Build history of the part. All positions in model axes, mm. Round coordinates to 2 decimals unless told otherwise and drop trailing zeros. Order: outer loops, then holes, each group sorted by start corner. A loop starts at its lowest first (then second) coordinate and runs counter-clockwise, first axis right, second up. Notation, with made-up numbers: M 8,39 L 37,39 A23 cw 37,58 Z; hole C 13.25,54.5 d11. An arc over 180 degrees is marked long. Use CSV: the item, a comma, the result in double quotes.
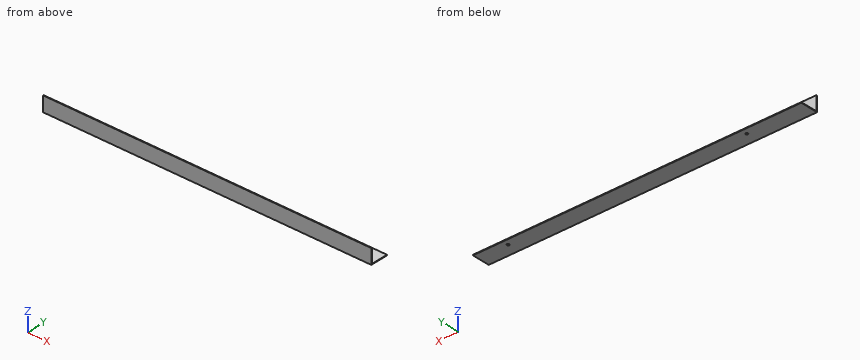
from build123d import *

# Parameters (mm, degrees)
F0_W     = 550
F0_H     = 30
F1_DEPTH = 1
F2_W     = 550
F2_H     = 1
F3_DEPTH = 24
F4_R     = 2
F5_DEPTH = 1.001


with BuildPart() as f1:
    # F0 (on Top) → F1 (new body)
    with BuildSketch(Plane.XY):
        with Locations((275, 15)):
            Rectangle(F0_W, F0_H)
    extrude(amount=F1_DEPTH)

    # F2 (on face) → F3 (join)
    with BuildSketch(Plane.XY.offset(1)):
        with Locations((275, 0.5)):
            Rectangle(F2_W, F2_H)
    extrude(amount=F3_DEPTH)

    # F4 (on face) → F5 (cut, through all)
    with BuildSketch(Plane.XY.offset(1)):
        with Locations((100, 20)):
            Circle(F4_R)
        with Locations((500, 20)):
            Circle(F4_R)
    extrude(amount=-F5_DEPTH, mode=Mode.SUBTRACT)


solid = f1.part
(1) Cut at B-B, the plane z = 14.75. Give the cut face in (x, y), and give its area (3 significant figures).
Answer block:
outline,"M 0,0 L 550,0 L 550,1 L 0,1 Z"
area,"550 mm²"
(2) Drop flat-ended pins along their axis: pin 1 (14.5 mm diameter, centred on x = 403, y = 16, fed in from +Z); pin 2 (2 mm diameter, centred on x = 271.5, z = 5.5, fed in from +Y). Give the stop position or say it passes through.
Answer block:
pin 1,"stops at z = 1"
pin 2,"stops at y = 1"
(3) Cut at A-A, the plane x = 188.5. Give the cut face in (y, z), and give its area (3 significant figures).
Answer block:
outline,"M 0,0 L 30,0 L 30,1 L 1,1 L 1,25 L 0,25 Z"
area,"54.0 mm²"
(4) Wall check: line 1 (Y direction, x = 100, z = 0.25); line 2 (Y direction, x = 235.5, z = 10.75). Give the ranges that are in metal, low to high. Write a range as from..to.
Answer block:
line 1,"y = 0..18, 22..30"
line 2,"y = 0..1"
